Can you work these out from the model? Positions are in its coordinate system, mm. Face numbers are marked on the shaded views. Round coordinates to 2 decimals unless told otherwise and drop trailing zeros. Loops run counter-clockwise (first coordinate to the right, second up) from the corner with the lowest first, then second, coordinate; pieces in that order, holes last. Notation, with made-up numbers: (55.5, 50.25) -> (70.5, 50.25) arc R16 ccw to (70.5, 54.25) -> close; hole circle Ø9 at (64.5, -1). An arc over 180 degrees is marked (long way). Write each question's results on one line, items separated by ' | '.
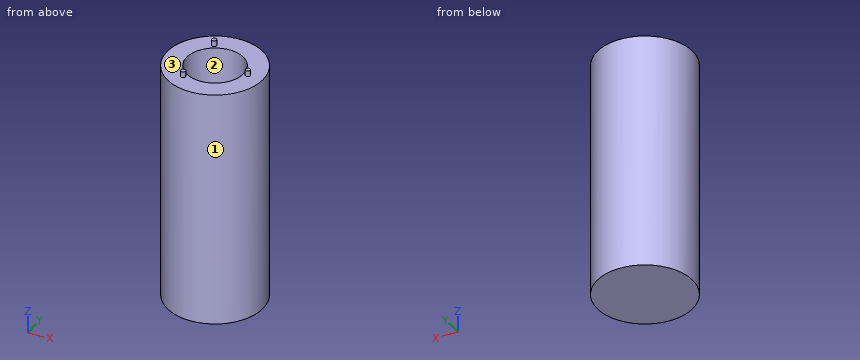
from build123d import *

# Parameters (mm, degrees)
F0_R     = 80
F0_R_2   = 4
F0_R_3   = 47.5
F1_DEPTH = 400
F2_DEPTH = 9.9
F3_DEPTH = 350


with BuildPart() as f1:
    # F0 (on Top) → F1 (new body)
    with BuildSketch(Plane.XY):
        Circle(F0_R)
        with Locations((-27.5, -47.631397)):
            Circle(F0_R_2, mode=Mode.SUBTRACT)
        with Locations((-27.5, 47.631397)):
            Circle(F0_R_2, mode=Mode.SUBTRACT)
        Circle(F0_R_3, mode=Mode.SUBTRACT)
        with Locations((55, 0)):
            Circle(F0_R_2, mode=Mode.SUBTRACT)
        Circle(F0_R_3)
        with Locations((-27.5, 47.631397)):
            Circle(F0_R_2)
        with Locations((55, 0)):
            Circle(F0_R_2)
        with Locations((-27.5, -47.631397)):
            Circle(F0_R_2)
    extrude(amount=-F1_DEPTH)

    # F0 (on Top) → F2 (join)
    with BuildSketch(Plane.XY):
        with Locations((-27.5, -47.631397)):
            Circle(F0_R_2)
        with Locations((55, 0)):
            Circle(F0_R_2)
        with Locations((-27.5, 47.631397)):
            Circle(F0_R_2)
    extrude(amount=F2_DEPTH)

    # F0 (on Top) → F3 (cut)
    with BuildSketch(Plane.XY):
        Circle(F0_R_3)
    extrude(amount=-F3_DEPTH, mode=Mode.SUBTRACT)


solid = f1.part
1. If we section it at A-A (y = 0): List the corners of the cut face in (x, z) for me, then the cut area to 3 significant figures.
Final values:
outline: (-80, -400) -> (80, -400) -> (80, 0) -> (59, 0) -> (59, 9.9) -> (51, 9.9) -> (51, 0) -> (47.5, 0) -> (47.5, -350) -> (-47.5, -350) -> (-47.5, 0) -> (-80, 0) -> close | area: 30,800 mm2
2. Please list where these lines run through material, in increasing order: line 1 (Y direction, x = 0, z = -71); line 2 (Z direction, x = 42, y = 17); line 3 (Z direction, x = 19, y = 62.5). Write a range as from..to.
Final values:
line 1: -80..-47.5, 47.5..80 | line 2: -400..-350 | line 3: -400..0
3. If we section it at C-C (z = -92): List the corners of the cut face in (x, y) for me, then the cut area to 3 significant figures.
Final values:
outline: circle Ø160 at (0, 0); hole circle Ø95 at (0, 0) | area: 13,000 mm2
4. We'd pull the mould along X, two halves only. Please class the marked faces 1, 2 and 3: pulls with the +X half, pulls with the -X half, needs draft (parallel to the pull), parting line crosses it, or undercut.
Final values:
face 1: parting line crosses it | face 2: undercut | face 3: needs draft
5. If we section it at D-D (x = 0): List the corners of the cut face in (y, z) for me.
Final values:
outline: (-80, -400) -> (80, -400) -> (80, 0) -> (47.5, 0) -> (47.5, -350) -> (-47.5, -350) -> (-47.5, 0) -> (-80, 0) -> close
6. Will these pins go through, and if not, where does the flat tip stop? pin 1 (3 mm diameter, centred on x = -16.5, z = -142, fed in from +Y); pin 2 (1.5 mm diameter, centred on x = -40.5, y = -17.5, fed in from +Z); pin 3 (6 mm diameter, centred on x = -1.5, z = -271.5, fed in from +Y).
Final values:
pin 1: y = 78.58 | pin 2: z = -350 | pin 3: y = 80
7. If we section it at B-B (x = 36.5): List the corners of the cut face in (y, z) for me.
Final values:
outline: (-71.19, -400) -> (71.19, -400) -> (71.19, 0) -> (30.4, 0) -> (30.4, -350) -> (-30.4, -350) -> (-30.4, 0) -> (-71.19, 0) -> close
